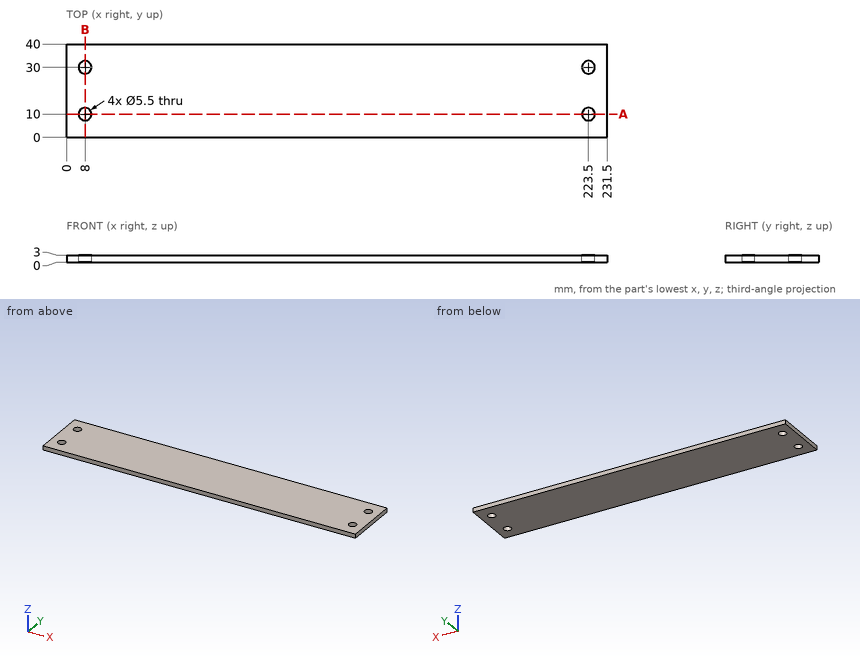
For this review, use the dimensioned drawing (mm, ordinates from the lowest corner) and the shaded views. Give positions to 0.01 mm unless a question says otherwise; leave off trailing zeros. Order: outer loops, then holes, each group sorted by start corner. A loop starts at its lowest first (then second) coordinate and runs counter-clockwise, first axis right, second up. Notation, with made-up numbers: M -9,-39 L 13,-39 A23 ccw 13,-7 Z; hole C -16.75,65 d6. An arc over 180 degrees is marked long. One line per question, with ' | ' between items. Start each with the question number.
1) Wall thickness on L1, parallel to Y at x = 223.5, z = 2.35; L2, parallel to X at y = 12.5, z = 0.9: over which ranges is each line inside the solid? List them lowest first. Write a range as from..to.
2) Consider section A-A, the plane y = 10. Give the boundary of the cut face in (x, z), then the cut area to 4 significant figures.
3) Consider section B-B, the plane x = 8. Give the boundary of the cut face in (y, z), then the cut area to 3 significant figures.
4) Clearance check with a flat-ended pin moving along its axis: P1, Ø9, axis at x = 8, y = 30, coming from the -Z side. State where the tip first meets the part, or that it passes through.
Found:
1) L1: y = 0..7.25, 12.75..27.25, 32.75..40 | L2: x = 0..6.85, 9.15..222.35, 224.65..231.5
2) outline: M 0,0 L 5.25,0 L 5.25,3 L 0,3 Z; M 10.75,0 L 220.75,0 L 220.75,3 L 10.75,3 Z; M 226.25,0 L 231.5,0 L 231.5,3 L 226.25,3 Z | area: 661.5 mm²
3) outline: M 0,0 L 7.25,0 L 7.25,3 L 0,3 Z; M 12.75,0 L 27.25,0 L 27.25,3 L 12.75,3 Z; M 32.75,0 L 40,0 L 40,3 L 32.75,3 Z | area: 87.0 mm²
4) P1: stops at z = 0
